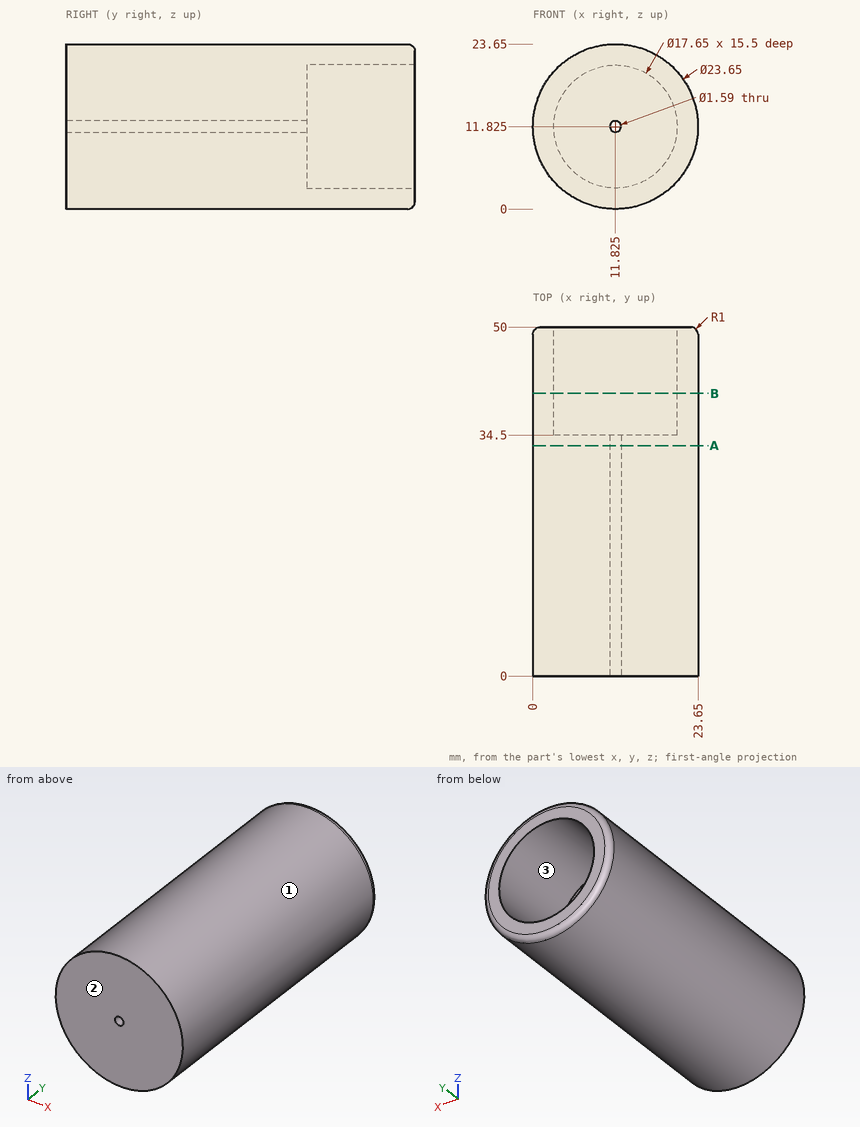
The figure shows three views and two pictorial views of one solid part (mm, origin at its lowest corner). Answer the questions. Give positions to 0.01 mm unless a question says otherwise; leave off trailing zeros. Loops run counter-clockwise (first coordinate to the right, second up) from the corner with the lowest first, then second, coordinate; pieces in that order, holes last. Notation, with made-up numbers: (21.25, 82.5) - (30.25, 82.5) arc R17 cw to (30.25, 109.5) - close; hole circle Ø7 at (-26, 22.5). An arc over 180 degrees is marked (long way). Use one line per item in the form item = value.
1. The mould has two halves that part along Z. Classify the marked faces 1, 2 and 3: pulls with the +Z half, pulls with the -Z half, needs draft (parallel to the pull), parting line crosses it, or undercut.
Calculated:
face_1 = parting line crosses it
face_2 = needs draft
face_3 = undercut
2. Find the intervals of material crossed by line 1 along Y through (x, z) = (14, 8.5); line 2 along Z through (x, y) = (11.75, 8); line 3 along X through (y, z) = (41, 17.75), in increasing order. Write a range as [from, to].
Calculated:
line_1 = [0, 34.5]
line_2 = [0, 11.03], [12.62, 23.65]
line_3 = [1.59, 5.28], [18.37, 22.06]
3. Section A-A on y = 33 is taken. Give the vertices of the cut face in (x, z) (3 decimals), then the cut area to 3 significant figures.
Calculated:
outline = circle Ø23.65 at (11.825, 11.825); hole circle Ø1.59 at (11.825, 11.825)
area = 437 mm^2
4. Section B-B on y = 40.5 is taken. Give the vertices of the cut face in (x, z) (3 decimals).
Calculated:
outline = circle Ø23.65 at (11.825, 11.825); hole circle Ø17.65 at (11.825, 11.825)
5. Given pin 1 Ø10 at (y, z) = (32, 2.5) entering from -X; pin 2 Ø12 at (x, y) = (20, 33.5) entering from +Z; pin 3 Ø1 at (x, z) = (15.5, 18) entering from +Y; pin 4 Ø1.4 at (x, z) = (11.825, 11.825) entering from +Y, each flat-ended and moving along its own axis, determine where each tip first touches the part or whether it passes through.
Calculated:
pin_1 = 0.82
pin_2 = 23.45
pin_3 = 34.5
pin_4 = through
